Autodesk Inventor part; units mm, degrees
ref_plane "Work Plane1" through (1.525, 0, 0) normal (0, 0, 1) x (1, 0, 0)
ref_plane "YZ Plane" through (0, 0, 0) normal (1, 0, 0) x (0, 1, 0)
ref_plane "XZ Plane" through (0, 0, 0) normal (0, 1, 0) x (-1, 0, 0)
sketch "Sketch1" plane through (0, 0, 0) normal (0, 0, 1) x (1, 0, 0)
  line L0 (0, 11.245) -> (0, 8)
  line L1 (6, 8) -> (55, 8)
  line L2 (55, 8) -> (55, 0)
  line L3 (55, 0) -> (-0.8001, 0)
  line L4 (-11.9601, 0) -> (66.16, 0)
  line L5 (-0.8001, 0) -> (-0.8001, 11.245)
  line L6 (-0.8001, 11.245) -> (0, 11.245)
  line L7 (6, 8) -> (4.773, 8)
  line L8 (4.773, 8) -> (0, 8)
  line L9 (0, -2.249) -> (0, 13.494)
  dimension "d0" = 55
  dimension "d1" = 49
  dimension "d2" = 16
  dimension "d9" = 0.8001
  dimension "d10" = 22.49
  dimension "d13" = 1.227
  dimension "d14" = 16
revolve "Body" add sketch "Sketch1" angle 360 about axis through (55, 0, 0) along (-1, 0, 0)
sketch "Sketch2" plane through (-0.8001, 0, 0) normal (-1, 0, 0) x (0, 0, 1)
  line L0 (0, 13.8564) -> (12, 6.9282)
  line L1 (12, 6.9282) -> (12, -6.9282)
  line L2 (12, -6.9282) -> (0, -13.8564)
  line L3 (0, -13.8564) -> (-12, -6.9282)
  line L4 (-12, -6.9282) -> (-12, 6.9282)
  line L5 (-12, 6.9282) -> (0, 13.8564)
  point P0 (0, 0)
  point P1 (0, 0)
  dimension "d11" = 24
extrude "Head" add sketch "Sketch2" along normal blind 9.2
sketch "Sketch4" plane through (0, 0, 0) normal (0, 0, 1) x (1, 0, 0)
  line L0 (-10.0001, 12) -> (-10.0001, 13.8564)
  line L1 (-10.0001, 13.8564) -> (-8.9283, 13.8564)
  line L2 (-8.9283, 13.8564) -> (-10.0001, 12)
  line L3 (-11.8401, 0) -> (1.0399, 0)
  line L4 (-0.8001, 13.8564) -> (-10.0001, 13.8564)
  line L5 (-10.0001, 6.9282) -> (-10.0001, 13.8564)
  dimension "d5" = 30
  dimension "d19" = 24
revolve "Chamfer1" cut sketch "Sketch4" angle 360 about axis through (-10, 0, 0) along (1, 0, 0)
thread "Thread"
chamfer "Chamfer2" distance 1.2269 distance2 1.227 1 edges at (55, -8, 0) measured on face at (55, -1.996, 1.7683)
ref_plane "Work Plane1" through (1.525, 0, 0) normal (0, 0, 1) x (1, 0, 0)
equation "\"d0\" = NLG"
equation "\"d1\" = GEL"
equation "\"d2\" = GD"
equation "\"d10\" = SD2"
equation "\"d14\" = BDM"
equation "\"d11\" = SW"
equation "\"d3\" = KOH - SD"
equation "\"d5\" = ANG1"
equation "\"d19\" = SW0"
equation "\"d15\" = GEL"
equation "\"d6\" = -0.5 * SPD + 0.5 * GD"
equation "\"NLG\" = 55"
equation "\"GD\" = NND"
equation "\"BDM\" = NND"
equation "\"KOH\" = 10"
equation "\"GEL\" = 49"
equation "\"SW\" = 24"
equation "\"SW0\" = SW"
equation "\"SPD\" = NND - 1.2269 * PTC"
equation "\"SD2\" = 22.49"
equation "\"SD\" = 0.8"
equation "\"ANG1\" = 30deg"
equation "\"GAL\" = 0.61345 * PTC"
equation "\"GUL\" = 0.61345 * PTC"
equation "\"RR\" = 0.6"
equation "\"GD1\" = THREADDIA - 1.2269 * PTC"
equation "\"THREADDIA\" = 16"
equation "\"SDH\" = SD2"
equation "\"SDHG\" = 6"
equation "\"TOA\" = 30deg"
equation "\"PTC\" = 2"
equation "\"NND\" = 16"
equation "\"E0\" = 27.72"
properties part number "ISO 4017 - M16 x 55" material "Stainless Steel, 440C"
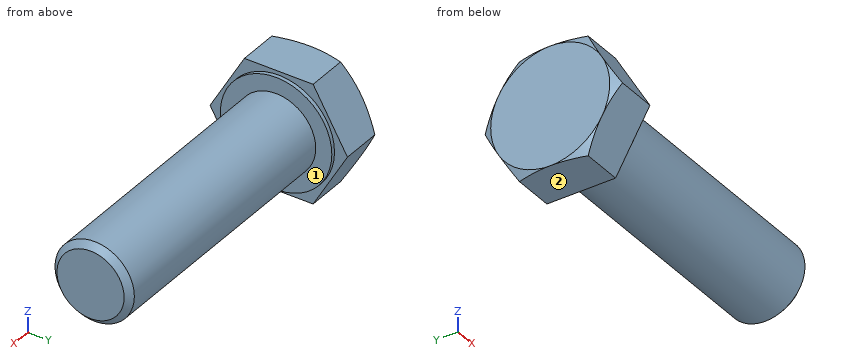
Model file for the job. Use its own axes, mm. Face numbers are marked on the shaded views. A direction names the side the tool comes from. Give positions to 0.01 mm unless a question says otherwise; leave off trailing zeros. Loops run counter-clockwise (first coordinate to the right, second up) from the corner with the lowest first, then second, coordinate; pieces in that order, holes last.
1) Saw through at A-A (x = 38). Write the cut outline in (y, z).
2) Tool access for the marked faces 1 and 2: list every direction of +Z, -Z, +X, -X, +Y, -Y with a clear straight run to the whole face (end or side of a thin tool).
3) Wall check: line 1 (Y direction, x = 31, z = 4); line 2 (X direction, y = -3.5, z = 9.25); line 3 (X direction, y = -5.5, z = -10). Give the ranges that are in metal, low to high.
4) Flat gauge pins, fed straight in: pin 1 Ø3 at (x, z) = (10.5, -2) entering from -Y; pin 2 Ø1.5 at (y, z) = (7.5, -4) entering from +X; pin 3 Ø6 at (x, z) = (29.5, -9) entering from -Y. Where does each tip first touch, or does it go through?
Answer block:
1. outline: circle Ø16 at (0, 0)
2. face 1: +X
2. face 2: -Z, +X, -X, +Y, -Y
3. line 1: y = -6.93 to 6.93
3. line 2: x = -10 to 0
3. line 3: x = -10 to -0.8
4. pin 1: stops at y = -7.98
4. pin 2: stops at x = 54.02
4. pin 3: stops at y = -5.29
